from build123d import *

# Parameters (mm, degrees)
SKETCH3_W           = 171.45
SKETCH3_H           = 127
BOSS_EXTRUDE1_DEPTH = 2.54
SKETCH4_W           = 2.54
SKETCH4_H           = 25.4
CUT_EXTRUDE1_DEPTH  = 3.54
LPATTERN1_COUNT     = 2
LPATTERN1_PITCH     = 50.8
SKETCH6_W           = 2.54
SKETCH6_H           = 25.4
CUT_EXTRUDE2_DEPTH  = 3.54
SKETCH7_W           = 2.54
SKETCH7_H           = 25.4
CUT_EXTRUDE3_DEPTH  = 3.54
SKETCH8_W           = 21.166666667
SKETCH8_H           = 2.54
CUT_EXTRUDE4_DEPTH  = 3.54
SKETCH9_R           = 11.43
CUT_EXTRUDE5_DEPTH  = 3.54
SKETCH10_R          = 3.175
CUT_EXTRUDE6_DEPTH  = 3.54
SKETCH11_R          = 1.27
CUT_EXTRUDE8_DEPTH  = 3.54
CIRPATTERN1_COUNT   = 4


with BuildPart() as part:
    # Sketch3 → Boss-Extrude1 (new body)
    with BuildSketch(Plane.XY):
        with Locations((85.725, 63.5)):
            Rectangle(SKETCH3_W, SKETCH3_H)
    extrude(amount=BOSS_EXTRUDE1_DEPTH)

    # Sketch4 → Cut-Extrude1 (cut, through all)
    with BuildSketch(Plane.XY.offset(2.54)):
        with Locations((1.27, 88.9)):
            Rectangle(SKETCH4_W, SKETCH4_H)
    cut_extrude1 = extrude(amount=-CUT_EXTRUDE1_DEPTH, mode=Mode.SUBTRACT)

    # LPattern1: Cut-Extrude1 ×2
    with Locations(*[(0, -i * LPATTERN1_PITCH, 0) for i in range(1, LPATTERN1_COUNT)]):
        add(cut_extrude1, mode=Mode.SUBTRACT)

    # Sketch6 → Cut-Extrude2 (cut, through all)
    with BuildSketch(Plane.XY.offset(2.54)):
        with Locations((170.18, 88.9)):
            Rectangle(SKETCH6_W, SKETCH6_H)
    extrude(amount=-CUT_EXTRUDE2_DEPTH, mode=Mode.SUBTRACT)

    # Sketch7 → Cut-Extrude3 (cut, through all)
    with BuildSketch(Plane.XY.offset(2.54)):
        with Locations((170.18, 38.1)):
            Rectangle(SKETCH7_W, SKETCH7_H)
    extrude(amount=-CUT_EXTRUDE3_DEPTH, mode=Mode.SUBTRACT)

    # Sketch8 → Cut-Extrude4 (cut, through all)
    with BuildSketch(Plane(origin=(0, 0, 0), x_dir=(-1, 0, 0), z_dir=(0, 0, -1))):
        with Locations((-38.184666667, 1.27)):
            Rectangle(SKETCH8_W, SKETCH8_H)
    extrude(amount=-CUT_EXTRUDE4_DEPTH, mode=Mode.SUBTRACT)

    # Sketch9 → Cut-Extrude5 (cut, through all)
    with BuildSketch(Plane(origin=(0, 0, 0), x_dir=(-1, 0, 0), z_dir=(0, 0, -1))):
        with Locations((-109.474, 63.5)):
            Circle(SKETCH9_R)
    extrude(amount=-CUT_EXTRUDE5_DEPTH, mode=Mode.SUBTRACT)

    # Sketch10 → Cut-Extrude6 (cut, through all)
    with BuildSketch(Plane(origin=(0, 0, 0), x_dir=(-1, 0, 0), z_dir=(0, 0, -1))):
        with Locations((-38.1, 63.5)):
            Circle(SKETCH10_R)
    extrude(amount=-CUT_EXTRUDE6_DEPTH, mode=Mode.SUBTRACT)

    # Sketch11 → Cut-Extrude8 (cut, through all)
    with BuildSketch(Plane(origin=(0, 0, 0), x_dir=(-1, 0, 0), z_dir=(0, 0, -1))):
        with Locations((-38.1, 73.025)):
            Circle(SKETCH11_R)
    cut_extrude8 = extrude(amount=-CUT_EXTRUDE8_DEPTH, mode=Mode.SUBTRACT)

    # CirPattern1: Cut-Extrude8 ×4 about axis
    cirpattern1_axis = Axis((38.1, 63.5, 0), (0, 0, 1))
    for i in range(1, CIRPATTERN1_COUNT):
        add(cut_extrude8.rotate(cirpattern1_axis, i * 360 / CIRPATTERN1_COUNT), mode=Mode.SUBTRACT)


solid = part.part
Check sheet for the modelled part. Datum: model origin and axes. Units: mm. Round coordinates to 2 decimals unless told otherwise and drop trailing zeros. Loops run counter-clockwise (first coordinate to the right, second up) from the corner with the lowest first, then second, coordinate; pieces in that order, holes last. Notation, with made-up numbers: M 63,33.25 L 100,33.25 A35 cw 100,70.25 Z; hole C 72.5,14.25 d5. An arc over 180 degrees is marked long. One line per item, written item: value.
(1) Sectioned sample at B-B, the plane z = 1.15. Count the separate pieces of the cut face and the enclosed holes in it, then the cut area to 3 significant figures.
Computed values:
separate pieces: 1
enclosed holes: 6
area: 21,000 mm^2
(2) Thickness scan on line 1 (Y direction, x = 38.1, z = 0.55) (3 decimals); line 2 (X direction, y = 97, z = 0.4); line 3 (X direction, y = 53, z = 0.5). Record the ranges inside material, lowest first.
Computed values:
line 1: y = 2.54 to 52.705, 55.245 to 60.325, 66.675 to 71.755, 74.295 to 127
line 2: x = 2.54 to 168.91
line 3: x = 0 to 37.29, 38.91 to 104.96, 113.99 to 171.45
(3) Release check for a two-part mould opening along X. For faces 1 (the face through (110.962, 74.833, 1.252)), 2 (the face through (85, 64, 2.54)), 3 (the face through (40.44, 65.646, 1.252)) record: +X half, -X half, draft (parallel to the pull), parting line (faces both ways), or undercut.
Computed values:
face 1: undercut
face 2: draft
face 3: undercut
(4) Sectioned sample at A-A, the plane y = 33.5. Record the cut outline in (x, z), then the cut area to 3 significant figures.
Computed values:
outline: M 2.54,0 L 168.91,0 L 168.91,2.54 L 2.54,2.54 Z
area: 423 mm^2
(5) Depth check by flat-ended pin: pin 1 Ø1.3 at (y, z) = (33.5, 1) entering from +X; pin 2 Ø2 at (x, y) = (38.1, 73.025) entering from +Z. Enter the tip coordinate at first touch or a pass-through.
Computed values:
pin 1: stops at x = 168.91
pin 2: passes through
